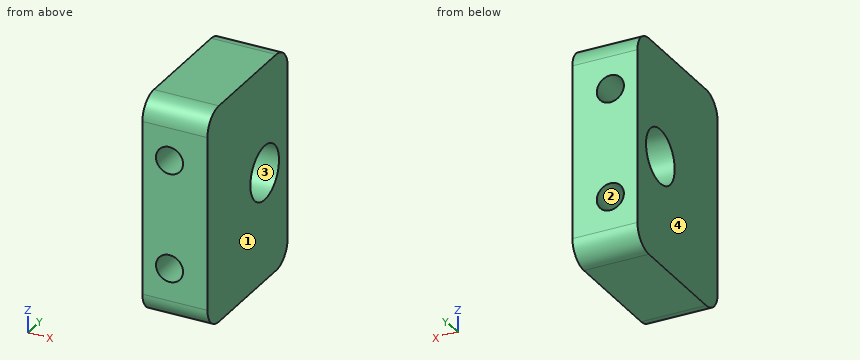
```python
from build123d import *

# Parameters (mm, degrees)
SKETCH_1_W          = 6
SKETCH_1_H          = 20
EXTRUDE_1_DEPTH     = 14
SKETCH_2_R          = 1.25
CUT_EXTRUDE_1_DEPTH = 14
SKETCH_3_R          = 2.5
CUT_EXTRUDE_2_DEPTH = 14
FILLET_1_R          = 2


with BuildPart() as part:
    # 草图1 → 凸台-拉伸1 (new body)
    with BuildSketch(Plane(origin=(0, 0, 0), x_dir=(1, 0, 0), z_dir=(0, 1, 0))):
        Rectangle(SKETCH_1_W, SKETCH_1_H)
    extrude(amount=EXTRUDE_1_DEPTH)

    # 草图2 → 切除-拉伸1 (cut)
    with BuildSketch(Plane(origin=(0, 14, 0), x_dir=(1, 0, 0), z_dir=(0, 1, 0))):
        with Locations(Location((-0.5, -5, 0), (0, 0, 270))):
            Circle(SKETCH_2_R)
        with Locations(Location((-0.5, 5, 0), (0, 0, 270))):
            Circle(SKETCH_2_R)
    extrude(amount=-CUT_EXTRUDE_1_DEPTH, mode=Mode.SUBTRACT)

    # 草图3 → 切除-拉伸2 (cut)
    with BuildSketch(Plane.ZY.offset(3)):
        with Locations((0, 10)):
            Circle(SKETCH_3_R)
    extrude(amount=-CUT_EXTRUDE_2_DEPTH, mode=Mode.SUBTRACT)

    # 圆角1
    fillet_1_edges = [part.edges().sort_by_distance(p)[0] for p in [
        (0, 14, 10),
        (0, 0, 10),
        (0, 0, -10),
        (0, 14, -10),
    ]]
    fillet(fillet_1_edges, radius=FILLET_1_R)


solid = part.part
```
Part model, mm, in its own coordinate system. Face numbers are marked on the shaded views. Round coordinates to 2 decimals unless told otherwise and drop trailing zeros. Loops run counter-clockwise (first coordinate to the right, second up) from the corner with the lowest first, then second, coordinate; pieces in that order, holes last.
1. Drill centre lines: line 1 along Z through (x, y) = (-0.45, 4.5); line 2 along Z through (x, y) = (-1.5, 9); line 3 along Z through (x, y) = (-0.45, 1.5). Where is each one in solid material? Low to high.
Solutions:
line 1: z = -10 to -6.25, -3.75 to 3.75, 6.25 to 10
line 2: z = -10 to -5.75, -4.25 to -2.29, 2.29 to 4.25, 5.75 to 10
line 3: z = -9.94 to -6.25, -3.75 to 3.75, 6.25 to 9.94
2. Slice it at D-D (x = 1.85). Give the cut face in (y, z), and give its area (3 significant figures).
Solutions:
outline: (0, -8) arc R2 ccw to (2, -10) - (12, -10) arc R2 ccw to (14, -8) - (14, 8) arc R2 ccw to (12, 10) - (2, 10) arc R2 ccw to (0, 8) - close; hole circle Ø5 at (10, 0)
area: 257 mm2
3. Slice it at B-B (z = 5). Give the cut face in (x, y), and give its area (3 significant figures).
Solutions:
outline: (-3, 0) - (-1.75, 0) - (-1.75, 14) - (-3, 14) - close; (0.75, 0) - (3, 0) - (3, 14) - (0.75, 14) - close
area: 49.0 mm2
4. Slice it at C-C (y = 10). Give the cut face in (x, z), and give its area (3 significant figures).
Solutions:
outline: (-3, -10) - (3, -10) - (3, -2.5) - (-3, -2.5) - close; (-3, 2.5) - (3, 2.5) - (3, 10) - (-3, 10) - close; hole circle Ø2.5 at (-0.5, -5); hole circle Ø2.5 at (-0.5, 5)
area: 80.2 mm2
5. Two-plate mould, pull along X, no slides. Class the marked faces 1, 2, 3 and 4: pulls with the +X half, pulls with the -X half, needs draft (parallel to the pull), parting line crosses it, or undercut.
Solutions:
face 1: pulls with the +X half
face 2: undercut
face 3: needs draft
face 4: pulls with the -X half
6. Slice it at A-A (x = -0.5). Give the cut face in (y, z).
Solutions:
outline: (0, -8) arc R2 ccw to (2, -10) - (12, -10) arc R2 ccw to (14, -8) - (14, -6.25) - (0, -6.25) - close; (0, -3.75) - (14, -3.75) - (14, 3.75) - (0, 3.75) - close; (0, 6.25) - (14, 6.25) - (14, 8) arc R2 ccw to (12, 10) - (2, 10) arc R2 ccw to (0, 8) - close; hole circle Ø5 at (10, 0)
